```python
from build123d import *

# Parameters (mm, degrees)
SKETCH1_R           = 35
BOSS_EXTRUDE1_DEPTH = 5


with BuildPart() as part:
    # Sketch1 → Boss-Extrude1 (new body)
    with BuildSketch(Plane(origin=(0, 0, 0), x_dir=(1, 0, 0), z_dir=(0, 1, 0))):
        Circle(SKETCH1_R)
        with BuildLine():
            Line((-1.4, 0.9), (-2.224859546, 0.9))
            ThreePointArc((-2.224859546, 0.9), (-2.4, 0), (-2.224859546, -0.9))
            Line((-2.224859546, -0.9), (-1.4, -0.9))
            ThreePointArc((-1.4, -0.9), (-1.046446609, -1.046446609), (-0.9, -1.4))
            Line((-0.9, -1.4), (-0.9, -2.224859546))
            ThreePointArc((-0.9, -2.224859546), (0, -2.4), (0.9, -2.224859546))
            Line((0.9, -2.224859546), (0.9, -1.4))
            ThreePointArc((0.9, -1.4), (1.046446609, -1.046446609), (1.4, -0.9))
            Line((1.4, -0.9), (2.224859546, -0.9))
            ThreePointArc((2.224859546, -0.9), (2.4, 0), (2.224859546, 0.9))
            Line((2.224859546, 0.9), (1.4, 0.9))
            ThreePointArc((1.4, 0.9), (1.046446609, 1.046446609), (0.9, 1.4))
            Line((0.9, 1.4), (0.9, 2.224859546))
            ThreePointArc((0.9, 2.224859546), (0, 2.4), (-0.9, 2.224859546))
            Line((-0.9, 2.224859546), (-0.9, 1.4))
            ThreePointArc((-0.9, 1.4), (-1.046446609, 1.046446609), (-1.4, 0.9))
        make_face(mode=Mode.SUBTRACT)
    extrude(amount=BOSS_EXTRUDE1_DEPTH)


solid = part.part
```
Check sheet for the modelled part. Datum: model origin and axes. Units: mm. A direction names the side the tool comes from. Give positions to 0.01 mm unless a question says otherwise; leave off trailing zeros. Loops run counter-clockwise (first coordinate to the right, second up) from the corner with the lowest first, then second, coordinate; pieces in that order, holes last. Notation, with made-up numbers: (23.5, 58) - (33.5, 58) arc R6 cw to (33.5, 66) - close; hole circle Ø6 at (-29.5, -14.75). An arc over 180 degrees is marked (long way). One line per question, with ' | ' between items. Start each with the question number.
1. Set-up check for faces 4 (the cylindrical face through (2.4, 2.5, 0)), 5 (the flat face through (0, 5, 7)): record each of +Z, -Z, +X, -X, +Y, -Y from which the full face is reachable in a straight line by a thin tool's end or side.
2. Cross-section at A-A, the plane y = 0.85. Enter the section's corners in (x, z).
3. Material ranges on line 1 along X through (y, z) = (3.7, -31.5); line 2 along X through (y, z) = (3.7, -29.5); line 3 along Z through (x, y) = (26, 1.85), recorded low to high. Write a range as [from, to].
4. Cross-section at D-D, the plane z = 21. Enter the section's corners in (x, y).
5. Cross-section at B-B, the plane x = 0. Enter the section's corners in (y, z).
6. Gauge pin test, flat ends, axial feed: pin 1 Ø0.7 at (x, y) = (-2, 3.5) entering from -Z; pin 2 Ø0.9 at (y, z) = (2, 2) entering from +X; pin 3 Ø0.7 at (y, z) = (3, -2) entering from -X; pin 4 Ø1.5 at (x, z) = (-11.5, 6) entering from -Y. Record the tip position at first contact, or that the pin passes through.
7. Cross-section at C-C, the plane z = 0. Enter the section's corners in (x, y).
8. Draft check along Z on faces 1 (the flat face through (0, 0, 7)), 2 (the cylindrical face through (-28, 2, 21)), 3 (the cylindrical face through (0, 2.5, -2.4)). Enter one of: released by +Z, released by -Z, zero draft, split by the parting line, or undercut.
Check result:
1) face 4: +Y, -Y | face 5: +Z, -Z, +X, -X, +Y
2) outline: circle Ø70 at (0, 0); hole (-2.22, -0.9) - (-1.4, -0.9) arc R0.5 cw to (-0.9, -1.4) - (-0.9, -2.22) arc R2.4 ccw to (0.9, -2.22) - (0.9, -1.4) arc R0.5 cw to (1.4, -0.9) - (2.22, -0.9) arc R2.4 ccw to (2.22, 0.9) - (1.4, 0.9) arc R0.5 cw to (0.9, 1.4) - (0.9, 2.22) arc R2.4 ccw to (-0.9, 2.22) - (-0.9, 1.4) arc R0.5 cw to (-1.4, 0.9) - (-2.22, 0.9) arc R2.4 ccw to start
3) line 1: x = [-15.26, 15.26] | line 2: x = [-18.83, 18.83] | line 3: z = [-23.43, 23.43]
4) outline: (-28, 0) - (28, 0) - (28, 5) - (-28, 5) - close
5) outline: (0, -35) - (5, -35) - (5, -2.4) - (0, -2.4) - close; (0, 2.4) - (5, 2.4) - (5, 35) - (0, 35) - close
6) pin 1: stops at z = -34.96 | pin 2: stops at x = 34.97 | pin 3: stops at x = -34.96 | pin 4: stops at y = 0
7) outline: (-35, 0) - (-2.4, 0) - (-2.4, 5) - (-35, 5) - close; (2.4, 0) - (35, 0) - (35, 5) - (2.4, 5) - close
8) face 1: zero draft | face 2: split by the parting line | face 3: undercut
